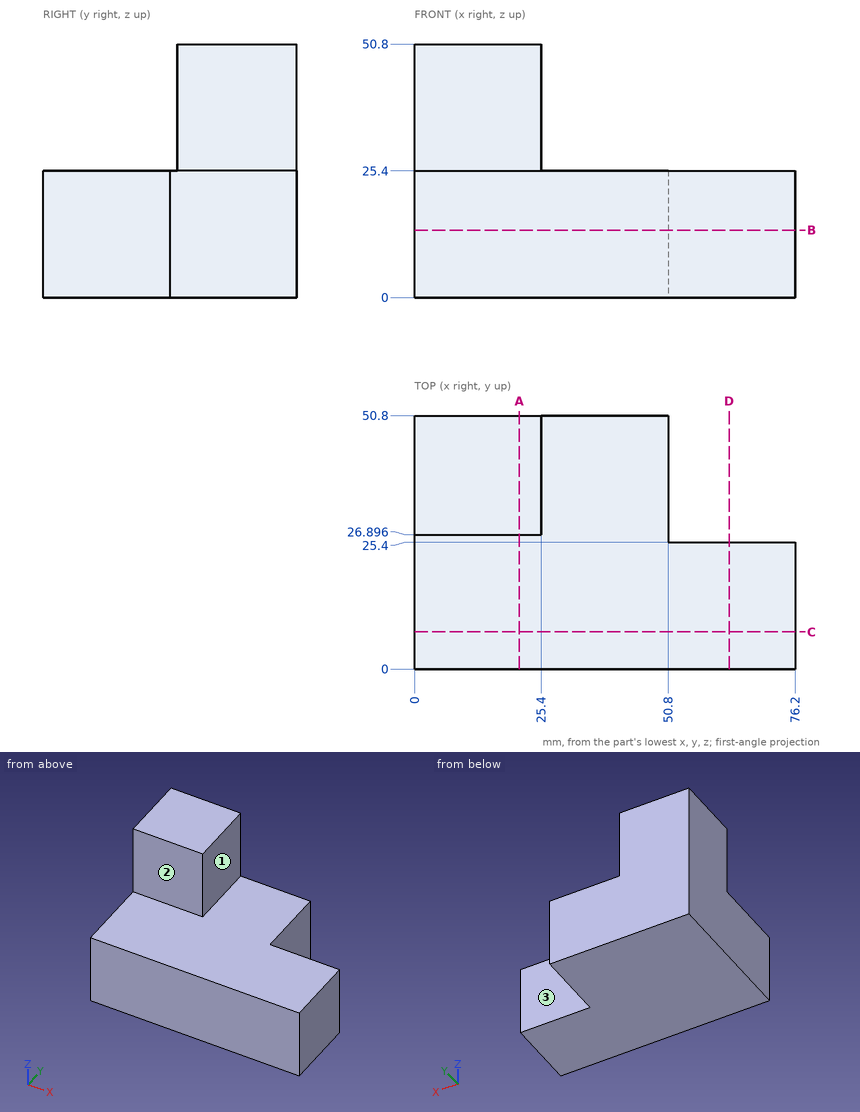
Study the drawing (mm; zero at the part's minimum x, y, z) and answer. A direction names the side the tool comes from. Give positions to 0.01 mm unless a question says otherwise; leave off trailing zeros. Loops run counter-clockwise (first coordinate to the right, second up) from the corner with the lowest first, then second, coordinate; pieces in that order, holes last. Notation, with made-up numbers: (-21.5, 3) - (-3.5, 3) arc R22 ccw to (-3.5, 13) - close; hole circle Ø10 at (-18.75, 70.25). An arc over 180 degrees is marked (long way). Use CSV: the item, a comma, the result in double quotes. Start each with the question number.
(1) Find section B-B, the plane z = 13.5. Determine the outline of the cut face in (x, y).
(2) Find section A-A, the plane x = 21. Determine the outline of the cut face in (y, z).
(3) A tool of negligible diameter and unlimited length cuts with its end or side. For the marked faces 1, 2 and 3, from which of +Z, -Z, +X, -X, +Y, -Y can it reach the whole face along a straight path? Write none if from no direction.
(4) Find section D-D, the plane x = 63. Determine the outline of the cut face in (y, z).
(5) Find section C-C, the plane y = 7.5. Determine the outline of the cut face in (x, z).
(6) Each of these flat-tipped pins is pushed along its axis until it touches: pin 1 (8 mm diameter, centred on x = 46, y = 23, fed in from -Z); pin 2 (19 mm diameter, centred on y = 37.5, z = 36, fed in from +X); pin 3 (1.5 mm diameter, centred on x = 12, z = 31.5, fed in from -Y); pin 4 (12 mm diameter, centred on x = 51.5, y = 21, fed in from +Z). Where does it stop, or does it pass through?
(7) Find the intervals of material crossed by L1, parallel to Z at x = 19, y = 13; L2, parallel to Y at x = 14, z = 31, in increasing order.
Results found:
1,outline,"(0, 0) - (76.2, 0) - (76.2, 25.4) - (50.8, 25.4) - (50.8, 50.8) - (0, 50.8) - close"
2,outline,"(0, 0) - (50.8, 0) - (50.8, 50.8) - (26.9, 50.8) - (26.9, 25.4) - (0, 25.4) - close"
3,face 1,"+Z, +X, +Y, -Y"
3,face 2,"+Z, +X, -X, -Y"
3,face 3,"+Z, -Z, +X, +Y"
4,outline,"(0, 0) - (25.4, 0) - (25.4, 25.4) - (0, 25.4) - close"
5,outline,"(0, 0) - (76.2, 0) - (76.2, 25.4) - (0, 25.4) - close"
6,pin 1,"z = 0"
6,pin 2,"x = 25.4"
6,pin 3,"y = 26.9"
6,pin 4,"z = 25.4"
7,L1,"0 to 25.4"
7,L2,"26.9 to 50.8"
